Here's how the part is built. I have some questions about the finished solid (model axes, mm). Give positions to 0.01 mm unless a question says otherwise; leave off trailing zeros. Loops run counter-clockwise (first coordinate to the right, second up) from the corner with the lowest first, then second, coordinate; pieces in that order, holes last. Notation, with made-up numbers: (8.5, 12.25) - (16.5, 12.25) arc R14 cw to (16.5, 25.25) - close; hole circle Ø9 at (-5.5, 6.25). An arc over 180 degrees is marked (long way). Use a Markdown table: item, result.
from build123d import *

# Parameters (mm, degrees)
SKETCH_1_W          = 20
SKETCH_1_H          = 20
SKETCH_1_W_2        = 17.6
SKETCH_1_H_2        = 17.6
EXTRUDE_1_DEPTH     = 280
SKETCH_2_W          = 20
SKETCH_2_H          = 10
CUT_EXTRUDE_1_DEPTH = 281.891438104
SKETCH_3_R          = 1.6
CUT_EXTRUDE_2_DEPTH = 281.891438104
CUT_EXTRUDE_3_REACH = 282.891
SKETCH_4_R          = 2.5


with BuildPart() as part:
    # 草图1 → 凸台-拉伸1 (new, symmetric)
    with BuildSketch(Plane(origin=(0, 0, 0), x_dir=(0, 0, -1), z_dir=(1, 0, 0))):
        Rectangle(SKETCH_1_W, SKETCH_1_H)
        Rectangle(SKETCH_1_W_2, SKETCH_1_H_2, mode=Mode.SUBTRACT)
    extrude(amount=EXTRUDE_1_DEPTH, both=True)

    # 草图2 → 切除-拉伸1 (cut, through all)
    with BuildSketch(Plane(origin=(0, 0, -10), x_dir=(-1, 0, 0), z_dir=(0, 0, -1))):
        with Locations((-85, 5)):
            Rectangle(SKETCH_2_W, SKETCH_2_H)
        with Locations((85, 5)):
            Rectangle(SKETCH_2_W, SKETCH_2_H)
    extrude(amount=-CUT_EXTRUDE_1_DEPTH, mode=Mode.SUBTRACT)

    # 草图3 → 切除-拉伸2 (cut, through all)
    with BuildSketch(Plane(origin=(0, 10, 0), x_dir=(1, 0, 0), z_dir=(0, 1, 0))):
        with Locations(Location((115, 0, 0), (0, 0, 270))):
            Circle(SKETCH_3_R)
        with Locations(Location((165, 0, 0), (0, 0, 270))):
            Circle(SKETCH_3_R)
        with Locations(Location((265, 0, 0), (0, 0, 270))):
            Circle(SKETCH_3_R)
        with Locations(Location((215, 0, 0), (0, 0, 270))):
            Circle(SKETCH_3_R)
        with Locations(Location((-215, 0, 0), (0, 0, 270))):
            Circle(SKETCH_3_R)
        with Locations(Location((-265, 0, 0), (0, 0, 270))):
            Circle(SKETCH_3_R)
        with Locations(Location((-115, 0, 0), (0, 0, 270))):
            Circle(SKETCH_3_R)
        with Locations(Location((-165, 0, 0), (0, 0, 270))):
            Circle(SKETCH_3_R)
    extrude(amount=-CUT_EXTRUDE_2_DEPTH, mode=Mode.SUBTRACT)

    # 草图4 → 切除-拉伸3 (cut, up to next)
    with BuildSketch(Plane.XZ.offset(10), mode=Mode.PRIVATE) as cut_extrude_3_sk1:
        with Locations(Location((240, 0, 0), (0, 0, 270))):
            Circle(SKETCH_4_R)
    cut_extrude_3_tool1 = extrude(cut_extrude_3_sk1.sketch, amount=-CUT_EXTRUDE_3_REACH, mode=Mode.PRIVATE) & part.part
    # 草图4 → 切除-拉伸3 (cut, up to next)
    with BuildSketch(Plane.XZ.offset(10), mode=Mode.PRIVATE) as cut_extrude_3_sk2:
        with Locations(Location((-240, 0, 0), (0, 0, 90))):
            Circle(SKETCH_4_R)
    cut_extrude_3_tool2 = extrude(cut_extrude_3_sk2.sketch, amount=-CUT_EXTRUDE_3_REACH, mode=Mode.PRIVATE) & part.part
    # 草图4 → 切除-拉伸3 (cut, up to next)
    with BuildSketch(Plane.XZ.offset(10), mode=Mode.PRIVATE) as cut_extrude_3_sk3:
        with Locations(Location((190, 0, 0), (0, 0, 270))):
            Circle(SKETCH_4_R)
    cut_extrude_3_tool3 = extrude(cut_extrude_3_sk3.sketch, amount=-CUT_EXTRUDE_3_REACH, mode=Mode.PRIVATE) & part.part
    # 草图4 → 切除-拉伸3 (cut, up to next)
    with BuildSketch(Plane.XZ.offset(10), mode=Mode.PRIVATE) as cut_extrude_3_sk4:
        with Locations(Location((140, 0, 0), (0, 0, 270))):
            Circle(SKETCH_4_R)
    cut_extrude_3_tool4 = extrude(cut_extrude_3_sk4.sketch, amount=-CUT_EXTRUDE_3_REACH, mode=Mode.PRIVATE) & part.part
    # 草图4 → 切除-拉伸3 (cut, up to next)
    with BuildSketch(Plane.XZ.offset(10), mode=Mode.PRIVATE) as cut_extrude_3_sk5:
        with Locations(Location((-140, 0, 0), (0, 0, 90))):
            Circle(SKETCH_4_R)
    cut_extrude_3_tool5 = extrude(cut_extrude_3_sk5.sketch, amount=-CUT_EXTRUDE_3_REACH, mode=Mode.PRIVATE) & part.part
    # 草图4 → 切除-拉伸3 (cut, up to next)
    with BuildSketch(Plane.XZ.offset(10), mode=Mode.PRIVATE) as cut_extrude_3_sk6:
        with Locations(Location((-190, 0, 0), (0, 0, 90))):
            Circle(SKETCH_4_R)
    cut_extrude_3_tool6 = extrude(cut_extrude_3_sk6.sketch, amount=-CUT_EXTRUDE_3_REACH, mode=Mode.PRIVATE) & part.part
    add(cut_extrude_3_tool1.solids().sort_by_distance((240, -10, 0))[0], mode=Mode.SUBTRACT)
    add(cut_extrude_3_tool2.solids().sort_by_distance((-240, -10, 0))[0], mode=Mode.SUBTRACT)
    add(cut_extrude_3_tool3.solids().sort_by_distance((190, -10, 0))[0], mode=Mode.SUBTRACT)
    add(cut_extrude_3_tool4.solids().sort_by_distance((140, -10, 0))[0], mode=Mode.SUBTRACT)
    add(cut_extrude_3_tool5.solids().sort_by_distance((-140, -10, 0))[0], mode=Mode.SUBTRACT)
    add(cut_extrude_3_tool6.solids().sort_by_distance((-190, -10, 0))[0], mode=Mode.SUBTRACT)


solid = part.part
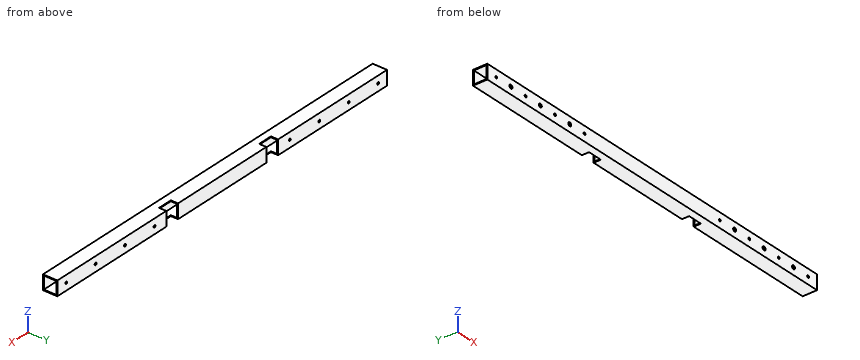
(1) Will this pin go through, and if not, where does the flat tip stop? pin 1 (5 mm diameter, centred on x = -89.5, z = -7, fed in from +Y).
A:
| item | result |
|---|---|
| pin 1 | y = 0 |
(2) If I drill on line 1 (Z direction, x = -179.5, y = 7.5); line 2 (Z direction, x = 115, y = 9.75), over which ranges is the centre line in solid material (lowest first)?
A:
| item | result |
|---|---|
| line 1 | -10 to -8.8, 8.8 to 10 |
| line 2 | -10 to -1.6, 1.6 to 10 |
(3) Suppose I cut it at A-A on y = 5.5. Write out the boundary of the cut face in (x, z).
A:
| item | result |
|---|---|
| outline | (-280, -10) - (-95, -10) - (-95, -8.8) - (-280, -8.8) - close; (-280, 8.8) - (-95, 8.8) - (-95, 10) - (-280, 10) - close; (-75, -10) - (75, -10) - (75, -8.8) - (-75, -8.8) - close; (-75, 8.8) - (75, 8.8) - (75, 10) - (-75, 10) - close; (95, -10) - (280, -10) - (280, -8.8) - (95, -8.8) - close; (95, 8.8) - (280, 8.8) - (280, 10) - (95, 10) - close |
(4) Suppose I cut it at B-B on x = 129. Write out the boundary of the cut face in (y, z).
A:
| item | result |
|---|---|
| outline | (-10, -10) - (10, -10) - (10, 10) - (-10, 10) - close; hole (-8.8, -8.8) - (8.8, -8.8) - (8.8, 8.8) - (-8.8, 8.8) - close |
